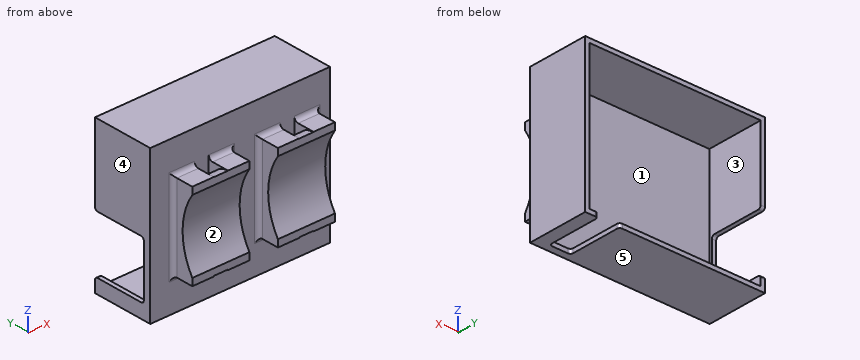
from build123d import *

# Parameters (mm, degrees)
SKETCH1_W           = 126
SKETCH1_H           = 106
SKETCH1_W_2         = 120
SKETCH1_H_2         = 100
BOSS_EXTRUDE1_DEPTH = 40
SKETCH5_W           = 126
SKETCH5_H           = 106
BOSS_EXTRUDE3_DEPTH = 3
SKETCH6_W           = 40
SKETCH6_H           = 60
BOSS_EXTRUDE4_DEPTH = 15
CUT_EXTRUDE3_DEPTH  = 92
SKETCH9_W           = 5
SKETCH9_H           = 3
CUT_EXTRUDE4_DEPTH  = 92
FILLET2_SIZE        = 15
FILLET2_SIZE_2      = 20
FILLET3_R           = 3
LPATTERN2_START     = -47
LPATTERN2_DEPTH     = 40
LPATTERN2_START_2   = -50
LPATTERN2_2_DEPTH   = 18
LPATTERN2_START_3   = -22
LPATTERN2_3_DEPTH   = 18
LPATTERN2_START_4   = -34
LPATTERN2_4_DEPTH   = 68
SKETCH10_W          = 15
SKETCH10_H          = 38
CUT_EXTRUDE5_DEPTH  = 10
SKETCH11_W          = 40
SKETCH11_H          = 38
CUT_EXTRUDE6_DEPTH  = 10
FILLET4_R           = 2


with BuildPart() as part:
    # Sketch1 → Boss-Extrude1 (new body)
    with BuildSketch(Plane(origin=(0, 0, 0), x_dir=(1, 0, 0), z_dir=(0, 1, 0))):
        Rectangle(SKETCH1_W, SKETCH1_H)
        Rectangle(SKETCH1_W_2, SKETCH1_H_2, mode=Mode.SUBTRACT)
    extrude(amount=BOSS_EXTRUDE1_DEPTH)

    # Sketch5 → Boss-Extrude3 (add)
    with BuildSketch(Plane.XZ):
        Rectangle(SKETCH5_W, SKETCH5_H)
    extrude(amount=BOSS_EXTRUDE3_DEPTH)

    # Sketch6 → Boss-Extrude4 (add)
    with BuildSketch(Plane.XZ.offset(3)):
        with Locations((33, 0)):
            Rectangle(SKETCH6_W, SKETCH6_H)
    extrude(amount=BOSS_EXTRUDE4_DEPTH)

    # Sketch7 → Cut-Extrude3 (cut)
    with BuildSketch(Plane(origin=(53, 0, 0), x_dir=(0, 0, -1), z_dir=(1, 0, 0))):
        with BuildLine():
            Line((-25, -18), (25, -18))
            ThreePointArc((25, -18), (0, -10.416573868), (-25, -18))
        make_face()
    extrude(amount=-CUT_EXTRUDE3_DEPTH, mode=Mode.SUBTRACT)

    # Sketch9 → Cut-Extrude4 (cut)
    with BuildSketch(Plane.XY.offset(30)):
        with Locations((30.5, -4.5)):
            Rectangle(SKETCH9_W, SKETCH9_H)
        with Locations((35.5, -4.5)):
            Rectangle(SKETCH9_W, SKETCH9_H)
    extrude(amount=-CUT_EXTRUDE4_DEPTH, mode=Mode.SUBTRACT)

    # Fillet2
    # a fillet whose section is not a circle: 20, 15 mm, written as the material it takes off along each edge
    with BuildSketch(Plane(origin=(38, -6, -30), x_dir=(0, 0, 1), z_dir=(-1, 0, 0))) as fillet2_piece_1:
        with BuildLine():
            Bezier((FILLET2_SIZE, 0), (0, 0), (0, -FILLET2_SIZE_2), weights=[1, 1.5, 1])
            Line((0, -FILLET2_SIZE_2), (0, 0))
            Line((0, 0), (FILLET2_SIZE, 0))
        make_face()
    extrude(amount=10, mode=Mode.SUBTRACT)
    with BuildSketch(Plane(origin=(28, -6, 30), x_dir=(0, 0, -1), z_dir=(1, 0, 0))) as fillet2_piece_2:
        with BuildLine():
            Bezier((FILLET2_SIZE_2, 0), (0, 0), (0, -FILLET2_SIZE), weights=[1, 1.5, 1])
            Line((0, -FILLET2_SIZE), (0, 0))
            Line((0, 0), (FILLET2_SIZE_2, 0))
        make_face()
    extrude(amount=10, mode=Mode.SUBTRACT)

    # Fillet3
    fillet3_edges = [part.edges().sort_by_distance(p)[0] for p in [
        (53, -3, 0),
        (45.5, -3, 30),
        (13, -3, 0),
        (20.5, -3, -30),
        (45.5, -3, -30),
        (20.5, -3, 30),
    ]]
    fillet(fillet3_edges, radius=FILLET3_R)



with BuildPart() as body_2:
    # LPattern2: read off the stored shape, not the designer's step
    # LPattern2 outline → LPattern2 (new body)
    with BuildSketch(Plane.YZ.offset(LPATTERN2_START)):
        with BuildLine():
            Line((-6, -15), (-6, 10))
            add(Edge.make_bspline(
                [(-6, 10), (-6, 28.973665961), (-18, 29.894663844)],
                knots=[0, 0, 0, 0.924950591, 0.924950591, 0.924950591], degree=2, weights=[1, 1.462475296, 1.069416995]))
            Line((-18, 29.894663844), (-18, 25))
            ThreePointArc((-18, 25), (-10.416573868, 0), (-18, -25))
            Line((-18, -25), (-18, -29.611278447))
            add(Edge.make_bspline(
                [(-18, -29.611278447), (-6, -28.174650985), (-6, -15)],
                knots=[0.172065577, 0.172065577, 0.172065577, 1, 1, 1], degree=2, weights=[1.142459014, 1.413967211, 1]))
        make_face()
    extrude(amount=LPATTERN2_DEPTH)


with BuildPart() as part_1:
    add(part.part)

    add(body_2.part)  # LPattern2 2 merges body 2
    # LPattern2 2 outline → LPattern2 2 (add)
    with BuildSketch(Plane.YZ.offset(LPATTERN2_START_2)):
        with BuildLine():
            ThreePointArc((-3, 33), (-3.878679656, 30.878679656), (-6, 30))
            Line((-6, 30), (-18, 30))
            Line((-18, 30), (-18, 29.894663844))
            add(Edge.make_bspline(
                [(-6, 10), (-6, 28.973665961), (-18, 29.894663844)],
                knots=[0, 0, 0, 0.924950591, 0.924950591, 0.924950591], degree=2, weights=[1, 1.462475296, 1.069416995]))
            Line((-6, 10), (-6, -15))
            add(Edge.make_bspline(
                [(-18, -29.611278447), (-6, -28.174650985), (-6, -15)],
                knots=[0.172065577, 0.172065577, 0.172065577, 1, 1, 1], degree=2, weights=[1.142459014, 1.413967211, 1]))
            Line((-18, -29.611278447), (-18, -30))
            Line((-18, -30), (-6, -30))
            ThreePointArc((-6, -30), (-3.878679656, -30.878679656), (-3, -33))
            Line((-3, -33), (-3, 33))
        make_face()
    extrude(amount=LPATTERN2_2_DEPTH)

    # LPattern2 3 outline → LPattern2 3 (add)
    with BuildSketch(Plane.YZ.offset(LPATTERN2_START_3)):
        with BuildLine():
            ThreePointArc((-3, 33), (-3.878679656, 30.878679656), (-6, 30))
            Line((-6, 30), (-18, 30))
            Line((-18, 30), (-18, 29.894663844))
            add(Edge.make_bspline(
                [(-6, 10), (-6, 28.973665961), (-18, 29.894663844)],
                knots=[0, 0, 0, 0.924950591, 0.924950591, 0.924950591], degree=2, weights=[1, 1.462475296, 1.069416995]))
            Line((-6, 10), (-6, -15))
            add(Edge.make_bspline(
                [(-18, -29.611278447), (-6, -28.174650985), (-6, -15)],
                knots=[0.172065577, 0.172065577, 0.172065577, 1, 1, 1], degree=2, weights=[1.142459014, 1.413967211, 1]))
            Line((-18, -29.611278447), (-18, -30))
            Line((-18, -30), (-6, -30))
            ThreePointArc((-6, -30), (-3.878679656, -30.878679656), (-3, -33))
            Line((-3, -33), (-3, 33))
        make_face()
    extrude(amount=LPATTERN2_3_DEPTH)

    # LPattern2 4 outline → LPattern2 4 (cut)
    with BuildSketch(Plane.XY.offset(LPATTERN2_START_4)):
        with BuildLine():
            Line((-50, -18), (-47, -18))
            Line((-47, -18), (-47, -6))
            ThreePointArc((-47, -6), (-47.878679656, -3.878679656), (-50, -3))
            Line((-50, -3), (-50, -18))
        make_face()
        with BuildLine():
            Line((-4, -18), (-4, -3))
            ThreePointArc((-4, -3), (-6.121320344, -3.878679656), (-7, -6))
            Line((-7, -6), (-7, -18))
            Line((-7, -18), (-4, -18))
        make_face()
    extrude(amount=LPATTERN2_4_DEPTH, mode=Mode.SUBTRACT)

    # Sketch10 → Cut-Extrude5 (cut)
    with BuildSketch(Plane(origin=(0, 0, -53), x_dir=(-1, 0, 0), z_dir=(0, 0, -1))):
        with Locations((-46.5, 21)):
            Rectangle(SKETCH10_W, SKETCH10_H)
    extrude(amount=-CUT_EXTRUDE5_DEPTH, mode=Mode.SUBTRACT)

    # Sketch11 → Cut-Extrude6 (cut)
    with BuildSketch(Plane.ZY.offset(63)):
        with Locations((-23, 21)):
            Rectangle(SKETCH11_W, SKETCH11_H)
    extrude(amount=-CUT_EXTRUDE6_DEPTH, mode=Mode.SUBTRACT)

    # Fillet4
    fillet4_edges = [part_1.edges().sort_by_distance(p)[0] for p in [
        (39, 40, -51.5),
        (54, 40, -51.5),
        (39, 2, -51.5),
        (54, 2, -51.5),
        (-61.5, 40, -3),
        (-61.5, 40, -43),
        (-61.5, 2, -3),
        (-61.5, 2, -43),
    ]]
    fillet(fillet4_edges, radius=FILLET4_R)


solid = part_1.part
CAD build for the part. Positions are in the model's coordinates, mm. Face numbers are marked on the shaded views. A direction names the side the tool comes from. Give positions to 0.01 mm unless a question says otherwise; leave off trailing zeros. Loops run counter-clockwise (first coordinate to the right, second up) from the corner with the lowest first, then second, coordinate; pieces in that order, holes last. Notation, with made-up numbers: M -21.5,-3.5 L 35.5,-3.5 A27 ccw 35.5,18.5 Z; hole C 83,-3 d11. An arc over 180 degrees is marked long. Answer in a Markdown table with one row per item. Add a question column.
Item 1: Band-saw the part on A-A on y = 31.5. Give the cut face in (x, z), then the cut area to 3 significant figures.
Item 2: Band-saw the part on C-C on z = 8. Give the cut face in (x, y).
Item 3: Band-saw the part on B-B on x = 45.5. Give the cut face in (y, z), then the cut area to 3 significant figures.
Item 4: Tool access for the marked faces 1 and 2: list every direction of +Z, -Z, +X, -X, +Y, -Y with a clear straight run to the whole face (end or side of a thin tool).
Item 5: Drop flat-ended pins along their axis: P1, Ø3.5, axis at x = -61, z = -21.5, coming from the +Y side; P2, Ø13, axis at x = -37, y = -11, coming from the +Z side; P3, Ø13, axis at x = -17, y = -13, coming from the -Z side. Give the stop position or say it passes through.
Item 6: Band-saw the part on D-D on z = 31.5. Give the cut face in (x, y), then the cut area to 3 significant figures.
Item 7: Probe probe 1 along X at (y, z) = (-7, -29.5); probe 2 along X at (y, z) = (27, 19); probe 3 along Z at (x, y) = (29.5, 34). List the from-to ranges inside material, lowest first.
Item 8: Mould opens along X. For the marked faces 3, 4 and 5 say: +X half, -X half, draft (parallel to the pull), parting line (faces both ways), or undercut.
Reply:
| question | item | result |
|---|---|---|
| 1 | outline | M -63,-53 L 39,-53 L 39,-50 L -60,-50 L -60,-43 L -63,-43 Z; M -63,-3 L -60,-3 L -60,50 L 60,50 L 60,-50 L 54,-50 L 54,-53 L 63,-53 L 63,53 L -63,53 Z |
| 1 | area | 1,190 mm^2 |
| 2 | outline | M -63,-3 L -50,-3 A3 cw -47,-6 L -47,-11.13 L -7,-11.13 L -7,-6 A3 cw -4,-3 L 10,-3 A3 cw 13,-6 L 13,-11.13 L 53,-11.13 L 53,-6 A3 cw 56,-3 L 63,-3 L 63,40 L 60,40 L 60,0 L -60,0 L -60,40 L -63,40 Z; hole M -32,-6 L -22,-6 L -22,-3 L -32,-3 Z; hole M 28,-6 L 38,-6 L 38,-3 L 28,-3 Z |
| 3 | outline | M -18,-30 L -6,-30 A3 cw -3,-33 L -3,-53 L 2,-53 L 2,-50 L 0,-50 L 0,50 L 40,50 L 40,53 L -3,53 L -3,33 A3 cw -6,30 L -18,30 L -18,25 A45 cw -18,-25 Z |
| 3 | area | 1,090 mm^2 |
| 4 | face 1 | +Y |
| 4 | face 2 | +X, -X, -Y |
| 5 | P1 | stops at y = 2 |
| 5 | P2 | stops at z = 30.4 |
| 5 | P3 | stops at z = -30 |
| 6 | outline | M -63,-3 L -50,-3 A3 cw -48.5,-3.4 L -32,-3.4 L -32,-3 L -22,-3 L -22,-3.4 L -5.5,-3.4 A3 cw -4,-3 L 10,-3 A3 cw 11.5,-3.4 L 28,-3.4 L 28,-3 L 38,-3 L 38,-3.4 L 54.5,-3.4 A3 cw 56,-3 L 63,-3 L 63,40 L 60,40 L 60,0 L -60,0 L -60,40 L -63,40 Z |
| 6 | area | 645 mm^2 |
| 7 | probe 1 | x = -47 to -32, -22 to -7, 13 to 28, 38 to 53 |
| 7 | probe 2 | x = -63 to -60, 60 to 63 |
| 7 | probe 3 | z = -53 to -50, 50 to 53 |
| 8 | face 3 | undercut |
| 8 | face 4 | -X half |
| 8 | face 5 | draft |
